```python
from build123d import *

# Parameters (mm, degrees)
SALIENTE_EXTRUIR1_DEPTH = 2.5
CROQUIS2_R              = 4.5
CROQUIS2_R_2            = 2.75
SALIENTE_EXTRUIR2_DEPTH = 3
CORTAR_EXTRUIR1_REACH   = 7.5
CROQUIS3_R              = 1.5
CROQUIS4_R              = 2.8
CORTAR_EXTRUIR2_DEPTH   = 1
CROQUIS5_R              = 4.5
CROQUIS5_R_2            = 3.5
CORTAR_EXTRUIR3_DEPTH   = 0.5
REDONDEO1_R             = 0.3


with BuildPart() as part:
    # Croquis1 → Saliente-Extruir1 (new body)
    with BuildSketch(Plane(origin=(0, 0, 0), x_dir=(1, 0, 0), z_dir=(0, 1, 0))):
        with BuildLine():
            Line((16.885625022, 2.722828188), (4.337337893, 4.5))
            ThreePointArc((4.337337893, 4.5), (-0.003678449, 6.249998918), (-4.342631854, 4.494891387))
            Line((-4.342631854, 4.494891387), (-16.854847994, 2.722828188))
            ThreePointArc((-16.854847994, 2.722828188), (-19.219222971, 0), (-16.854847994, -2.722828188))
            Line((-16.854847994, -2.722828188), (-4.342631854, -4.494891387))
            ThreePointArc((-4.342631854, -4.494891387), (-0.003678449, -6.249998918), (4.337337893, -4.5))
            Line((4.337337893, -4.5), (16.885625022, -2.722828188))
            ThreePointArc((16.885625022, -2.722828188), (19.25, 0), (16.885625022, 2.722828188))
        make_face()
    extrude(amount=SALIENTE_EXTRUIR1_DEPTH)

    # Croquis2 → Saliente-Extruir2 (add)
    with BuildSketch(Plane(origin=(0, 2.5, 0), x_dir=(1, 0, 0), z_dir=(0, 1, 0))):
        Circle(CROQUIS2_R)
        Circle(CROQUIS2_R_2, mode=Mode.SUBTRACT)
    extrude(amount=SALIENTE_EXTRUIR2_DEPTH)

    # Croquis3 → Cortar-Extruir1 (cut, up to next)
    with BuildSketch(Plane.XZ, mode=Mode.PRIVATE) as cortar_extruir1_sk1:
        Circle(CROQUIS3_R)
    cortar_extruir1_tool1 = extrude(cortar_extruir1_sk1.sketch, amount=-CORTAR_EXTRUIR1_REACH, mode=Mode.PRIVATE) & part.part
    add(cortar_extruir1_tool1.solids().sort_by_distance((0, 0, 0))[0], mode=Mode.SUBTRACT)

    # Croquis4 → Cortar-Extruir2 (cut)
    with BuildSketch(Plane.XZ):
        Circle(CROQUIS4_R)
    extrude(amount=-CORTAR_EXTRUIR2_DEPTH, mode=Mode.SUBTRACT)

    # Croquis5 → Cortar-Extruir3 (cut)
    with BuildSketch(Plane.XZ):
        Circle(CROQUIS5_R)
        Circle(CROQUIS5_R_2, mode=Mode.SUBTRACT)
    extrude(amount=-CORTAR_EXTRUIR3_DEPTH, mode=Mode.SUBTRACT)

    # Redondeo1
    redondeo1_edges = [part.edges().sort_by_distance(p)[0] for p in [
        (-4.5, 5.5, 0),
        (-2.75, 5.5, 0),
        (-2.8, 0, 0),
        (-4.5, 0, 0),
        (-3.5, 0, 0),
    ]]
    fillet(redondeo1_edges, radius=REDONDEO1_R)


solid = part.part
```
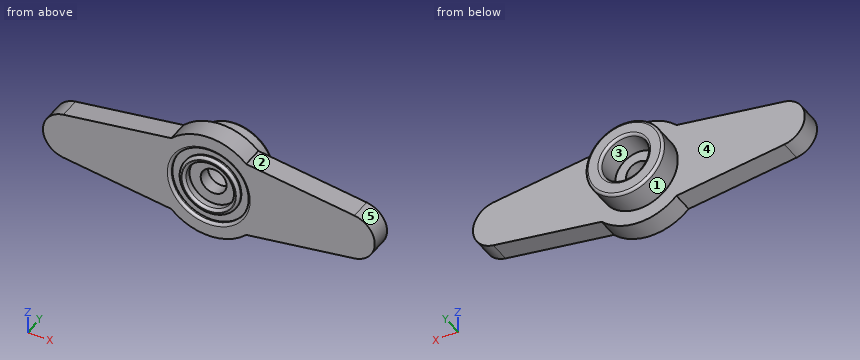
Here's how the part is built. I have some questions about the finished solid (model axes, mm). Face numbers are marked on the shaded views. A direction names the side the tool comes from. Give positions to 0.01 mm unless a question says otherwise; leave off trailing zeros. Loops run counter-clockwise (first coordinate to the right, second up) from the corner with the lowest first, then second, coordinate; pieces in that order, holes last. Notation, with made-up numbers: (-14.75, 84.25) -> (40.25, 84.25) arc R18 cw to (40.25, 115.25) -> close; hole circle Ø7 at (41.25, -1.75). An arc over 180 degrees is marked (long way). Use one line per item in the form item = value. Start each with the question number.
1) Which directions (+Z, -Z, +X, -X, +Y, -Y) give clear straight access to the entire face, cutting with the end or side of a thin tool? Please do the marked faces 1 and 2.
2) Imagine slicing it at A-A (y = 4.4). Please give me the cut outline in (x, z).
3) Thinking about a two-plate mould opening in Z: for the marked faces 3, 4 and 5, which applies, +Z half, -Z half, draft (parallel to the pull), parting line (faces both ways), or undercut?
4) Please list where these lines run through material, in increasing order: line 1 along X through (y, z) = (4.5, 0); line 2 along Y through (x, z) = (-2, -1.25); line 3 along Y through (x, z) = (9, -1.5).
5) For P1, Ø3.5, axis at x = 0, z = 0, coming from the -Y side; P2, Ø5, axis at x = 0, z = 0, coming from the +Y side; P3, Ø3, axis at x = -4, y = 1, coming from the +Z side, each with a flat end and sliding along its axis, tell me the tip position at first contact or that it passes through.
6) Imagine slicing it at B-B (x = -6). Please give me the cut outline in (y, z).
7) Imagine slicing it at C-C (z = -5.25). Please give me the cut outline in (x, y).
Check values:
q1.face_1 = +Y
q1.face_2 = +Z, +X, +Y, -Y
q2.outline = circle Ø9 at (0, 0); hole circle Ø5.5 at (0, 0)
q3.face_3 = undercut
q3.face_4 = draft
q3.face_5 = parting line
q4.line_1 = -4.5 to -2.75, 2.75 to 4.5
q4.line_2 = 1 to 2.5
q4.line_3 = 0 to 2.5
q5.P1 = 1
q5.P2 = 2.5
q5.P3 = 5.73
q6.outline = (0, -4.26) -> (2.5, -4.26) -> (2.5, 4.26) -> (0, 4.26) -> close
q7.outline = (-3.39, 0) -> (3.39, 0) -> (3.39, 2.5) -> (-3.39, 2.5) -> close
